Autodesk Inventor part; units mm, degrees
ref_plane "YZ Plane" through (0, 0, 0) normal (1, 0, 0) x (0, 1, 0)
ref_plane "XZ Plane" through (0, 0, 0) normal (0, 1, 0) x (-1, 0, 0)
ref_plane "XY Plane" through (0, 0, 0) normal (0, 0, 1) x (1, 0, 0)
sketch "スケッチ1" plane through (0, 0, 0) normal (0, 1, 0) x (-1, 0, 0)
  line L0 (-0.3902, 0.2385) -> (-82.3902, 0.2385)
  line L1 (-82.3902, 0.2385) -> (-82.3902, 30.2385)
  line L2 (-82.3902, 30.2385) -> (-0.3902, 30.2385)
  line L3 (-0.3902, 30.2385) -> (-0.3902, 0.2385)
  point P0 (0, 0)
  dimension "d0" = 82
  dimension "d1" = 30
extrude "押し出し1" add sketch "スケッチ1" along normal blind 5
sketch "スケッチ2" plane through (0, 5, 0) normal (0, 1, 0) x (1, 0, 0)
  line L0 (82.3902, -0.2385) -> (0.3902, -0.2385)
  line L1 (0.3902, -30.2385) -> (82.3902, -30.2385)
  line L2 (0.3902, -0.2385) -> (3.3902, -0.2385)
  line L3 (3.3902, -0.2385) -> (3.3902, -30.2385)
  line L4 (3.3902, -30.2385) -> (0.3902, -30.2385)
  line L5 (0.3902, -30.2385) -> (0.3902, -0.2385)
  line L6 (82.3902, -30.2385) -> (79.3902, -30.2385)
  line L7 (79.3902, -30.2385) -> (79.3902, -0.2385)
  line L8 (79.3902, -0.2385) -> (82.3902, -0.2385)
  line L9 (82.3902, -0.2385) -> (82.3902, -30.2385)
  point P0 (0, 0)
  dimension "d4" = 3
  dimension "d5" = 3
extrude "押し出し2" add sketch "スケッチ2" along normal blind 100 contours L9 L1 L7 L0 | L3 L1 L5 L0
properties part number "知能ロボコン大砲５"
Input: part model. Units: mm. Frame: model coordinates. A direction names the side the tool comes from. Give positions to 0.01 mm unless a question says otherwise; leave off trailing zeros. Loops run counter-clockwise (first coordinate to the right, second up) from the corner with the lowest first, then second, coordinate; pieces in that order, holes last. Notation, with made-up numbers: M 47,-19 L 76,-19 A24 cw 76,4 Z; hole C 49,50.25 d6. An arc over 180 degrees is marked long. Use one line per item in the form item = value.
1. Pull-direction query (X, two-part tool) for faces 3 (the face through (3.39, 54, 15)), 4 (the face through (82.39, 52, 15)), 5 (the face through (42, 0, 15)); classes: released by +X, released by -X, zero draft, split by the parting line, or undercut.
Numbers:
face_3 = undercut
face_4 = released by +X
face_5 = zero draft
2. Line query: L1, parallel to X at y = 6.5, z = 12; L2, parallel to Y at x = 6, z = 19.5. Output: solid intervals per line, ascending.
Numbers:
L1 = 0.39 to 3.39, 79.39 to 82.39
L2 = 0 to 5
3. Reachability of faces 1 (the face through (0.39, 52, 15)), 2 (the face through (79.39, 54, 15)) from +Z, -Z, +X, -X, +Y, -Y: full face, straight path, thin tool, end or side. Return the list, or none.
Numbers:
face_1 = +Z, -Z, -X, +Y, -Y
face_2 = +Z, -Z, +Y
4. Section query B-B, the plane z = 8.5. Return the cut outline in (x, y), and give its area (3 significant figures).
Numbers:
outline = M 0.39,0 L 82.39,0 L 82.39,105 L 79.39,105 L 79.39,5 L 3.39,5 L 3.39,105 L 0.39,105 Z
area = 1,010 mm²
5. Section query C-C, the plane x = 47. Return the cut outline in (y, z), and give its area (3 significant figures).
Numbers:
outline = M 0,0.24 L 5,0.24 L 5,30.24 L 0,30.24 Z
area = 150 mm²
6. First-contact query: pin 1 (1.5 mm diameter, centred on x = 16, z = 8, fed in from +Y). Flat tip, straight axial feed; report the tip coordinate or a pass-through.
Numbers:
pin_1 = 5
7. Section query A-A, the plane y = 41.5. Return the cut outline in (x, z), and give its area (3 significant figures).
Numbers:
outline = M 0.39,0.24 L 3.39,0.24 L 3.39,30.24 L 0.39,30.24 Z; M 79.39,0.24 L 82.39,0.24 L 82.39,30.24 L 79.39,30.24 Z
area = 180 mm²
